```python
from build123d import *

# Parameters (mm, degrees)
SKETCH1_R               = 7.5
BOSS_EXTRUDE1_DEPTH     = 1.95
BOSS_EXTRUDE2_DEPTH     = 5
BOSS_EXTRUDE3_DEPTH     = 40
BOSS_EXTRUDE5_DEPTH     = 2.5
SKETCH20_W              = 10
SKETCH20_H              = 3.999999996
BOSS_EXTRUDE6_DEPTH     = 2.5
BOSS_EXTRUDE7_DEPTH     = 2.5
CUT_EXTRUDE8_DEPTH      = 42.5
CUT_EXTRUDE9_DEPTH      = 42.5
CUT_EXTRUDE9_DEPTH_BACK = 42.5
SKETCH25_R              = 3.5
BOSS_EXTRUDE8_DEPTH     = 2
SKETCH26_R              = 3.5
BOSS_EXTRUDE9_DEPTH     = 2
SKETCH27_R              = 6
BOSS_EXTRUDE10_DEPTH    = 12.25
SKETCH33_R              = 25
SKETCH33_R_2            = 12.5
BOSS_EXTRUDE11_DEPTH    = 9.25
SKETCH40_R              = 12.5
BOSS_EXTRUDE13_DEPTH    = 2.5
BOSS_EXTRUDE12_REACH    = 34.5
SKETCH34_R              = 6
SKETCH47_R              = 14
SKETCH47_R_2            = 12.5
CUT_EXTRUDE10_DEPTH     = 0.1
SKETCH48_R              = 14
SKETCH48_R_2            = 12.5
CUT_EXTRUDE13_DEPTH     = 0.1


with BuildPart() as part:
    # Sketch1 → Boss-Extrude1 (new body)
    with BuildSketch(Plane.XY):
        with BuildLine():
            Line((-15.00003653, 25.228715134), (15.00003653, 25.228715134))
            Line((15.00003653, 25.228715134), (15.00003653, 13.228715134))
            ThreePointArc((15.00003653, 13.228715134), (0, -20), (-15.00003653, 13.228715134))
            Line((-15.00003653, 13.228715134), (-15.00003653, 25.228715134))
        make_face()
        Circle(SKETCH1_R, mode=Mode.SUBTRACT)
    extrude(amount=BOSS_EXTRUDE1_DEPTH)

    # Sketch4 → Boss-Extrude2 (add)
    with BuildSketch(Plane.XY.offset(1.95)):
        with BuildLine():
            Line((-12.50003653, 25.228715134), (-12.50003653, 12.247411431))
            ThreePointArc((-12.50003653, 12.247411431), (0, -17.5), (12.50003653, 12.247411431))
            Line((12.50003653, 12.247411431), (12.50003653, 25.228715134))
            Line((12.50003653, 25.228715134), (15.00003653, 25.228715134))
            Line((15.00003653, 25.228715134), (15.00003653, 13.228715134))
            ThreePointArc((15.00003653, 13.228715134), (0, -20), (-15.00003653, 13.228715134))
            Line((-15.00003653, 13.228715134), (-15.00003653, 25.228715134))
            Line((-15.00003653, 25.228715134), (-12.50003653, 25.228715134))
        make_face()
    extrude(amount=BOSS_EXTRUDE2_DEPTH)

    # Sketch7 → Boss-Extrude3 (add)
    with BuildSketch(Plane.XY.offset(6.95)):
        with BuildLine():
            Line((-17.320505157, -10.000005055), (-14.361403097, -10.000005055))
            ThreePointArc((-14.361403097, -10.000005055), (-17.439068776, 1.459068274), (-12.50003653, 12.247411431))
            Line((-12.50003653, 12.247411431), (-12.50003653, 15.612465749))
            Line((-12.50003653, 15.612465749), (-12.50003653, 25.228715134))
            Line((-12.50003653, 25.228715134), (-15.00003653, 25.228715134))
            Line((-15.00003653, 25.228715134), (-15.00003653, 13.228715134))
            ThreePointArc((-15.00003653, 13.228715134), (-19.900947569, 1.988035678), (-17.320505157, -10.000005055))
        make_face()
        with BuildLine():
            Line((17.320505157, -10.000005055), (14.361403097, -10.000005055))
            ThreePointArc((14.361403097, -10.000005055), (17.439068776, 1.459068274), (12.50003653, 12.247411431))
            Line((12.50003653, 12.247411431), (12.50003653, 15.612465749))
            Line((12.50003653, 15.612465749), (12.50003653, 25.228715134))
            Line((12.50003653, 25.228715134), (15.00003653, 25.228715134))
            Line((15.00003653, 25.228715134), (15.00003653, 13.228715134))
            ThreePointArc((15.00003653, 13.228715134), (19.900947569, 1.988035678), (17.320505157, -10.000005055))
        make_face()
    extrude(amount=BOSS_EXTRUDE3_DEPTH)

    # Sketch19 → Boss-Extrude5 (add)
    with BuildSketch(Plane(origin=(15.00003653, 0, 0), x_dir=(0, 0, -1), z_dir=(1, 0, 0))):
        Polygon((-36.95, 29.22871513), (0, 25.228715134), (-36.95, 25.228715134), align=None)
    extrude(amount=-BOSS_EXTRUDE5_DEPTH)

    # Sketch20 → Boss-Extrude6 (add)
    with BuildSketch(Plane(origin=(15.00003653, 0, 0), x_dir=(0, 0, -1), z_dir=(1, 0, 0))):
        with Locations((-41.95, 27.228715132)):
            Rectangle(SKETCH20_W, SKETCH20_H)
    extrude(amount=-BOSS_EXTRUDE6_DEPTH)

    # Sketch22 → Boss-Extrude7 (add)
    with BuildSketch(Plane.ZY.offset(15.00003653)):
        Polygon((46.95, 25.228715134), (46.95, 29.22871513), (36.95, 29.22871513), (0, 25.228715134), align=None)
    extrude(amount=-BOSS_EXTRUDE7_DEPTH)

    # Sketch10 → Cut-Extrude8 (cut)
    with BuildSketch(Plane(origin=(15.00003653, 0, 0), x_dir=(0, 0, -1), z_dir=(1, 0, 0))):
        with BuildLine():
            Line((-46.95, 25.228715134), (-46.95, 29.22871513))
            Line((-46.95, 29.22871513), (-36.95, 29.22871513))
            add(Edge.make_bspline(
                [(-36.95, 29.22871513), (-54.95, 21.22871513), (-36.95, 13.228715134)],
                knots=[0, 0, 0, 1, 1, 1], degree=2))
            Line((-36.95, 13.228715134), (-46.95, 13.228715134))
            Line((-46.95, 13.228715134), (-46.95, 25.228715134))
        make_face()
    extrude(amount=-CUT_EXTRUDE8_DEPTH, mode=Mode.SUBTRACT)

    # Sketch24 → Cut-Extrude9 (cut, two sides)
    with BuildSketch(Plane(origin=(15.00003653, 0, 0), x_dir=(0, 0, -1), z_dir=(1, 0, 0))) as cut_extrude9_sk:
        Polygon((-36.95, 13.228715134), (-6.95, -10.000005055), (-46.95, -10.000005055), (-46.95, 13.228715134), align=None)
    extrude(amount=CUT_EXTRUDE9_DEPTH, mode=Mode.SUBTRACT)
    extrude(cut_extrude9_sk.sketch, amount=-CUT_EXTRUDE9_DEPTH_BACK, mode=Mode.SUBTRACT)

    # Sketch25 → Boss-Extrude8 (add)
    with BuildSketch(Plane.ZY.offset(15.00003653)):
        with Locations((39.45, 21.22871513)):
            Circle(SKETCH25_R)
    extrude(amount=BOSS_EXTRUDE8_DEPTH)

    # Sketch26 → Boss-Extrude9 (add)
    with BuildSketch(Plane(origin=(15.00003653, 0, 0), x_dir=(0, 0, -1), z_dir=(1, 0, 0))):
        with Locations((-39.45, 21.22871513)):
            Circle(SKETCH26_R)
    extrude(amount=BOSS_EXTRUDE9_DEPTH)

    # Sketch27 → Boss-Extrude10 (add)
    with BuildSketch(Plane.ZY.offset(-12.50003653)):
        with Locations((38.7, 21.22871513)):
            Circle(SKETCH27_R)
    extrude(amount=BOSS_EXTRUDE10_DEPTH)



with BuildPart() as body_2:
    # Sketch33 → Boss-Extrude11 (new body, symmetric)
    with BuildSketch(Plane.ZY.offset(-0.25003653)):
        with Locations((38.7, 21.22871513)):
            Circle(SKETCH33_R)
        with Locations((38.7, 21.22871513)):
            Circle(SKETCH33_R_2, mode=Mode.SUBTRACT)
    extrude(amount=BOSS_EXTRUDE11_DEPTH, both=True)


with BuildPart() as part_1:
    add(part.part)

    add(body_2.part)  # Boss-Extrude13 merges body 2
    # Sketch40 → Boss-Extrude13 (add, symmetric)
    with BuildSketch(Plane.ZY.offset(-0.25003653)):
        with Locations((38.7, 21.22871513)):
            Circle(SKETCH40_R)
    extrude(amount=BOSS_EXTRUDE13_DEPTH, both=True)

    # Sketch34 → Boss-Extrude12 (add, up to next)
    with BuildSketch(Plane(origin=(-12.50003653, 0, 0), x_dir=(0, 0, -1), z_dir=(1, 0, 0)), mode=Mode.PRIVATE) as boss_extrude12_sk1:
        with Locations((-38.7, 21.22871513)):
            Circle(SKETCH34_R)
    boss_extrude12_tool1 = extrude(boss_extrude12_sk1.sketch, amount=BOSS_EXTRUDE12_REACH, mode=Mode.PRIVATE) - part_1.part
    add(boss_extrude12_tool1.solids().sort_by_distance((-12.500037, 21.228715, 38.7))[0])

    # Sketch47 → Cut-Extrude10 (cut)
    with BuildSketch(Plane.ZY.offset(8.99996347)):
        with Locations((38.7, 21.22871513)):
            Circle(SKETCH47_R)
        with Locations((38.7, 21.22871513)):
            Circle(SKETCH47_R_2, mode=Mode.SUBTRACT)
    extrude(amount=-CUT_EXTRUDE10_DEPTH, mode=Mode.SUBTRACT)

    # Sketch48 → Cut-Extrude13 (cut)
    with BuildSketch(Plane(origin=(9.50003653, 0, 0), x_dir=(0, 0, -1), z_dir=(1, 0, 0))):
        with Locations((-38.7, 21.22871513)):
            Circle(SKETCH48_R)
        with Locations((-38.7, 21.22871513)):
            Circle(SKETCH48_R_2, mode=Mode.SUBTRACT)
    extrude(amount=-CUT_EXTRUDE13_DEPTH, mode=Mode.SUBTRACT)


solid = part_1.part
```
Read the model definition and answer for the solid it produces. Units are mm, in the model's axes. A direction names the side the tool comes from. Give positions to 0.01 mm unless a question says otherwise; leave off trailing zeros. Write each loop counter-clockwise with the first axis right and the second up, starting at its lowest first coordinate (ties: lowest second). Pieces come first, ordered by that corner, then holes. Notation, with made-up numbers: (9.25, 30.25) -> (22.25, 30.25) arc R19 ccw to (22.25, 62.25) -> close; hole circle Ø5 at (30.25, 10). An arc over 180 degrees is marked (long way). Answer as a JSON object with one key per item and string values.
1) Section A-A on z = 30 is taken. Count the separate pieces of the cut face and the enclosed holes in it, then the cut area to 3 significant figures.
Findings below:
{"separate pieces": "3", "enclosed holes": "0", "area": "732 mm^2"}
2) A tool of negligible diameter and unlimited length cuts with its end or side. For faces 5 (the flat face through (-17.864, 1.777, 22.16)), 6 (the cylindrical face through (-5.5, 13.6, 28.8)), 7 (the flat face through (0, -18, 6.95)), from which of +Z, -Z, +X, -X, +Y, -Y can it reach the whole face along a straight path? Write none if from no direction.
Findings below:
{"face 5": "+Z, -X, -Y", "face 6": "none", "face 7": "+Z, +X, -X, -Y"}
3) Flat-ended cylindrical pins translate along their axes: pin 1 Ø12.5 at (y, z) = (17, 43.5) entering from +X; pin 2 Ø20 at (y, z) = (21.23, 38.7) entering from -X; pin 3 Ø6 at (y, z) = (36.5, 24) entering from -X; pin 4 Ø5 at (x, y) = (7.5, -4) entering from -Z. Find the tip coordinate at first contact, or state that the pin passes through.
Findings below:
{"pin 1": "stops at x = 17", "pin 2": "stops at x = -17", "pin 3": "stops at x = -9", "pin 4": "stops at z = 0"}
4) Straight lines are drawn through the part: probe 1 along Y at (x, z) = (3, 39); probe 2 along Z at (x, y) = (7, 15); probe 3 along Y at (x, z) = (0, 0.8). For each, find the intervals that lie inside material, in ascending order. Write a range as from..to.
Findings below:
{"probe 1": "y = -3.77..8.73, 15.24..27.22, 33.73..46.23", "probe 2": "z = 0..1.95, 14.49..27.86, 49.54..62.91", "probe 3": "y = -20..-7.5, 7.5..25.23"}
5) Section D-D on x = 4 is taken. Write down the section's boundary in (y, z).
Findings below:
{"outline": "(-19.6, 0) -> (-6.34, 0) -> (-6.34, 1.95) -> (-17.04, 1.95) -> (-17.04, 6.95) -> (-19.6, 6.95) -> close; circle Ø50 at (21.23, 38.7); (6.34, 0) -> (25.23, 0) -> (25.23, 1.95) -> (6.34, 1.95) -> close; circle Ø12 at (21.23, 38.7); hole circle Ø25 at (21.23, 38.7)"}
6) Section B-B on y = 0 is taken. Write down the section's boundary in (x, z).
Findings below:
{"outline": "(-20, 0) -> (-7.5, 0) -> (-7.5, 1.95) -> (-17.5, 1.95) -> (-17.5, 19.87) -> (-20, 19.87) -> close; (-9, 25.5) -> (9.5, 25.5) -> (9.5, 51.9) -> (-9, 51.9) -> close; (7.5, 0) -> (20, 0) -> (20, 19.87) -> (17.5, 19.87) -> (17.5, 1.95) -> (7.5, 1.95) -> close"}
7) Section C-C on x = 16 is taken. Write down the section's boundary in (y, z).
Findings below:
{"outline": "(-12, 0) -> (12, 0) -> (12, 35.36) -> (7.09, 29.02) -> (7.09, 1.95) -> (-7.09, 1.95) -> (-7.09, 10.71) -> (-10, 6.95) -> (-12, 6.95) -> close; circle Ø7 at (21.23, 39.45)"}
8) For a pull along Z with two mould halves and no side action, classify faces 1 (the cylindrical face through (-7.45, 15.37, 40)), 2 (the flat face through (15, 21, 22)), 3 (the flat face through (-13.768, 27.257, 18.734)), 4 (the cylindrical face through (6.1, 13.6, 28.8)) as pulls with the +Z half, pulls with the -Z half, needs draft (parallel to the pull), parting line crosses it, or undercut.
Findings below:
{"face 1": "undercut", "face 2": "needs draft", "face 3": "pulls with the -Z half", "face 4": "undercut"}
